from build123d import *

# Parameters (mm, degrees)
F0_W     = 67.1
F0_H     = 138.3
F1_DEPTH = 3.55
F2_T     = -2.54
F3_R     = 5.08
F4_W     = 20.894948
F4_H     = 9.035654
F5_DEPTH = 12.5
F6_W     = 8.791138
F6_H     = 3.129049
F7_DEPTH = 12.5


with BuildPart() as f1:
    # F0 (on Front) → F1 (new body, symmetric)
    with BuildSketch(Plane.XZ):
        Rectangle(F0_W, F0_H)
    extrude(amount=F1_DEPTH, both=True)

    # F2
    f2_openings = [f1.faces().sort_by_distance(p)[0] for p in [
        (0, -3.55, 0),
    ]]
    offset(amount=F2_T, openings=f2_openings)

    # F3
    f3_edges = [f1.edges().sort_by_distance(p)[0] for p in [
        (-33.55, 0, -69.15),
        (-33.55, 0, 69.15),
        (33.55, 0, 69.15),
        (33.55, 0, -69.15),
    ]]
    fillet(f3_edges, radius=F3_R)

    # F4 (on Front) → F5 (cut, symmetric)
    with BuildSketch(Plane.XZ):
        with Locations((17.661508, 60.631018)):
            Rectangle(F4_W, F4_H)
    extrude(amount=F5_DEPTH, both=True, mode=Mode.SUBTRACT)

    # F6 (on face) → F7 (cut, symmetric)
    with BuildSketch(Plane(origin=(0, 0, -69.15), x_dir=(1, 0, 0), z_dir=(0, 0, -1))):
        with Locations((0.192333, 0.072404)):
            Rectangle(F6_W, F6_H)
    extrude(amount=F7_DEPTH, both=True, mode=Mode.SUBTRACT)


solid = f1.part
Read the model definition and answer for the solid it produces. Units are mm, in the model's axes. A direction names the side the tool comes from. Give positions to 0.01 mm unless a question says otherwise; leave off trailing zeros. Write each loop counter-clockwise with the first axis right and the second up, starting at its lowest first coordinate (ties: lowest second). Pieces come first, ordered by that corner, then holes. Notation, with made-up numbers: (-25, 53.5) -> (4, 53.5) arc R35 ccw to (4, 85.5) -> close; hole circle Ø4 at (-22.5, -36). An arc over 180 degrees is marked (long way). Answer as a JSON object with one key per item and string values. Group by question number.
1) This flat-tipped pin is pushed along its axis until it touches: P1, Ø8, axis at x = -10, z = -17, coming from the -Y side. Where does it stop, or does it pass through?
2) Consider L1, parallel to X at y = 0.25, z = 52; L2, parallel to Z at x = 23, y = 3; L3, parallel to Z at x = 9, y = -1. Determine where each line is inside the solid, lowest interval first. Write a range as from..to.
3) The mould has two halves that part along X. Classify faces 1 (the cylindrical face through (32.101, -0.05, -67.622)), 2 (the flat face through (0, 3.55, 1)), 3 (the flat face through (4.588, 1.3, -65.7)): +X half, -X half, draft (parallel to the pull), parting line (faces both ways), or undercut.
4) Find section B-B (x = 18.5). Write down the section's boundary in (y, z), and give its area (3 significant figures).
5) Find section C-C (x = -9). Write down the section's boundary in (y, z), and give its area (3 significant figures).
6) A tool of negligible diameter and unlimited length cuts with its end or side. For faces 4 (the flat face through (0, 1.492, -63)), 5 (the flat face through (0, -2, -66.61)), 6 (the flat face through (18, 2, 56.113)), from which of +Z, -Z, +X, -X, +Y, -Y can it reach the whole face along a straight path? Write none if from no direction.
7) Find section A-A (z = 59.5). Write down the section's boundary in (x, y), and give its area (3 significant figures).
Values follow:
{
 "1": {"P1": "stops at y = 1.01"},
 "2": {"L1": "x = -33.55..-31.01, 31.01..33.55", "L2": "z = -69.15..56.11, 65.15..69.15", "L3": "z = -69.15..-66.61, 66.61..69.15"},
 "3": {"face 1": "+X half", "face 2": "draft", "face 3": "undercut"},
 "4": {"outline": "(-3.55, -69.15) -> (3.55, -69.15) -> (3.55, 56.11) -> (1.01, 56.11) -> (1.01, -66.61) -> (-3.55, -66.61) -> close; (-3.55, 66.61) -> (1.01, 66.61) -> (1.01, 65.15) -> (3.55, 65.15) -> (3.55, 69.15) -> (-3.55, 69.15) -> close", "area": "351 mm2"},
 "5": {"outline": "(-3.55, -69.15) -> (3.55, -69.15) -> (3.55, 69.15) -> (-3.55, 69.15) -> (-3.55, 66.61) -> (1.01, 66.61) -> (1.01, -66.61) -> (-3.55, -66.61) -> close", "area": "374 mm2"},
 "6": {"face 4": "-Z", "face 5": "-Y", "face 6": "+Y, -Y"},
 "7": {"outline": "(-33.55, -3.55) -> (-31.01, -3.55) -> (-31.01, 1.01) -> (7.21, 1.01) -> (7.21, 3.55) -> (-33.55, 3.55) -> close; (28.11, 1.01) -> (31.01, 1.01) -> (31.01, -3.55) -> (33.55, -3.55) -> (33.55, 3.55) -> (28.11, 3.55) -> close", "area": "141 mm2"}
}
